Geometry check sheet. Reference: the model listing, model coordinates, mm. A direction names the side the tool comes from. Round coordinates to 2 decimals unless told otherwise and drop trailing zeros. Loops run counter-clockwise (first coordinate to the right, second up) from the corner with the lowest first, then second, coordinate; pieces in that order, holes last. Notation, with made-up numbers: M 34,15.25 L 61,15.25 A23 ccw 61,25.25 Z; hole C 38,0.25 d8. An arc over 180 degrees is marked long. Answer in a Markdown table with one row per item. Add a question column.
Autodesk Fusion 360 part; units mm, degrees
sketch "Skizze1" plane through (0, 0, 0) normal (0, 0, 1) x (1, 0, 0)
  circle A0 centre (0, 0) radius 7.55
  line L0 (20, -10) -> (-10, -10)
  line L1 (-10, -10) -> (-10, 53.5)
  line L2 (-10, 53.5) -> (20, 53.5)
  line L3 (20, 53.5) -> (20, -10)
  line L4 (0, 0) -> (0, -10)
  line L5 (0, -10) -> (-0.5, -10)
  line L6 (-0.5, -10) -> (0.5, -10)
  line L7 (0.5, -10) -> (0.5, -7.3)
  line L8 (0.5, -7.3) -> (-0.5, -7.3)
  line L9 (-0.5, -7.3) -> (-0.5, -10)
  line L10 (-18, 3.5) -> (-18, -3.5)
  line L11 (-18, 3.5) -> (-18.5, 3.5)
  line L12 (-18, -3.5) -> (-18.5, -3.5)
  line L13 (-18.5, -3.5) -> (-18.5, -10)
  line L14 (-18.5, -10) -> (-10, -10)
  line L15 (-18.5, 3.5) -> (-18.5, 8.5)
  line L16 (-18.5, 8.5) -> (-10, 8.5)
  line L17 (-10, 53.5) -> (-20, 53.5)
  line L18 (-20, 53.5) -> (-20, 8.5)
  line L19 (-20, 8.5) -> (-10, 8.5)
  line L20 (-10, 8.5) -> (-10, 53.5)
  dimension "d1" = 15.1
  dimension "d4" = 20
  dimension "d5" = 10
  dimension "d6" = 10
  dimension "d7" = 63.5
  dimension "d15" = 18
  dimension "d16" = 7
  dimension "d17" = 3.5
  dimension "d18" = 0.5
  dimension "d19" = 0.5
  dimension "d54" = 10
extrude "Extrusion1" add sketch "Skizze1" along normal blind 50 contours A0 L0 L1 L2 L3 L7 L9 L20 | L1 L10 L11 L12 L13 L14 L15 L16 L19 | L1 L16 L17 L18 L19 L20
sketch "Skizze2" plane through (20, 0, 0) normal (1, 0, 0) x (0, 1, 0)
  line L0 (-10, 0) -> (53.5, 0)
  line L1 (53.5, 0) -> (53.5, 50)
  line L2 (53.5, 50) -> (-10, 50)
  line L3 (-10, 50) -> (-10, 0)
  circle A0 centre (0, 25) radius 4.15
  circle A1 centre (30, 25) radius 11.75
  line L4 (14.5, 40.5) -> (45.5, 40.5)
  line L5 (45.5, 40.5) -> (45.5, 9.5)
  line L6 (45.5, 9.5) -> (14.5, 9.5)
  line L7 (14.5, 9.5) -> (14.5, 40.5)
  circle A2 centre (14.5, 40.5) radius 3.25
  circle A3 centre (45.5, 40.5) radius 3.25
  circle A4 centre (45.5, 9.5) radius 3.25
  circle A5 centre (14.5, 9.5) radius 3.25
  circle A6 centre (14.5, 40.5) radius 1.75
  circle A7 centre (45.5, 40.5) radius 1.75
  circle A8 centre (45.5, 9.5) radius 1.75
  circle A9 centre (14.5, 9.5) radius 1.75
  circle A10 centre (0, 7.5) radius 4.15
  circle A11 centre (0, 42.5) radius 4.15
  dimension "d10" = 8.3
  dimension "d11" = 10
  dimension "d42" = 25
  dimension "d55" = 30
  dimension "d56" = 25
  dimension "d57" = 23.5
  dimension "d58" = 31
  dimension "d59" = 31
  dimension "d60" = 15.5
  dimension "d61" = 15.5
  dimension "d62" = 6.5
  dimension "d63" = 3.5
  dimension "d78" = 10
  dimension "d80" = 10
  dimension "d81" = 17.5
  dimension "d82" = 17.5
extrude "Extrusion7" cut sketch "Skizze2" against normal blind 40 contours A1 | L4 L7 A6 | L4 L7 A6 | L4 L5 A7 | L4 L5 A7 | L6 L7 A9 | L6 L7 A9 | L5 L6 A8 | L5 L6 A8
extrude "Extrusion8" cut sketch "Skizze2" against normal blind 35 contours L4 L7 A2 A6 | L4 L7 A2 A6 | L4 L5 A3 A7 | L4 L5 A3 A7 | L6 L7 A5 A9 | L6 L7 A5 A9 | L5 L6 A4 A8 | L5 L6 A4 A8
extrude "Extrusion2" cut sketch "Skizze2" against normal blind 11 contours A0 | A10 | A11
sketch "Skizze3" plane through (0, 0, 50) normal (0, 0, 1) x (-1, 0, 0)
  line L0 (18, -3.5) -> (18, 3.5)
  line L1 (18, 3.5) -> (18.5, 3.5)
  line L2 (18.5, 3.5) -> (18.5, 10)
  line L3 (18.5, 10) -> (10, 10)
  line L4 (10, 10) -> (0.5, 10)
  line L5 (0.5, 10) -> (0.5, 7.5334)
  arc A0 (-0.5, 7.5334) -> (0.5, 7.5334) centre (0, 0) ccw
  line L6 (-0.5, 7.5334) -> (-0.5, 10)
  line L7 (-0.5, 10) -> (-20, 10)
  line L8 (-20, 10) -> (-20, -53.5)
  line L9 (-20, -53.5) -> (20, -53.5)
  line L10 (18.5, -8.5) -> (18.5, -3.5)
  line L11 (18.5, -3.5) -> (18, -3.5)
  line L12 (-20, -53.5) -> (10, -53.5)
  line L13 (10, -53.5) -> (10, -8.5)
  line L14 (-20, -8.5) -> (-20, -53.5)
  arc A1 (-10, -8.5) -> (10, -8.5) centre (0, 0) ccw
  line L15 (-10, -8.5) -> (-20, -8.5)
  line L16 (20, -53.5) -> (20, -8.5)
  line L17 (20, -8.5) -> (18.5, -8.5)
sketch "Skizze5" plane through (0, 53.5, 0) normal (0, 1, 0) x (-1, 0, 0)
  line L0 (-20, 50) -> (-20, 0)
  line L1 (-20, 0) -> (20, 0)
  line L2 (-20, 25) -> (-13, 25)
  line L3 (-13, 25) -> (-13, 29.75)
  line L4 (-13, 25) -> (-13, 20.25)
  circle A0 centre (-13, 29.75) radius 1.15
  circle A1 centre (-13, 20.25) radius 1.15
  line L5 (20, 50) -> (-20, 50)
  line L6 (20, 0) -> (20, 50)
  dimension "d23" = 7
  dimension "d24" = 4.75
  dimension "d25" = 2.3
  dimension "d26" = 2.3
extrude "Extrusion4" cut sketch "Skizze5" against normal blind 11 contours A0 | A1
sketch "Skizze6" plane through (-18.5, 0, 0) normal (-1, 0, 0) x (0, -1, 0)
  line L0 (-8.5, 0) -> (-3.5, 0)
  line L1 (-3.5, 0) -> (-3.5, 50)
  line L2 (-3.5, 50) -> (-8.5, 50)
  line L3 (-6, 50) -> (-6, 0)
  line L4 (6, 50) -> (6, 0)
  circle A0 centre (-6, 42.5) radius 1.5
  circle A1 centre (-6, 7.5) radius 1.5
  circle A2 centre (6, 7.5) radius 1.5
  circle A3 centre (6, 42.5) radius 1.5
  line L5 (3.5, 50) -> (10, 50)
  line L6 (3.5, 0) -> (10, 0)
  line L7 (-8.5, 50) -> (-8.5, 0)
  circle A4 centre (-6, 42.5) radius 3.25
  circle A5 centre (-6, 7.5) radius 3.25
  dimension "d29" = 12
  dimension "d30" = 3
  dimension "d31" = 3
  dimension "d32" = 3
  dimension "d33" = 3
  dimension "d35" = 7.5
  dimension "d36" = 7.5
  dimension "d37" = 7.5
  dimension "d38" = 7.5
  dimension "d73" = 6.5
  dimension "d74" = 6.5
extrude "Extrusion5" cut sketch "Skizze6" against normal blind 7 contours L3 A1 | L3 A1 | L3 A0 | L3 A0 | L4 A3 | L4 A2 | L4 A2 | L4 A3
sketch "Skizze9" plane through (0, 53.5, 0) normal (0, 1, 0) x (-1, 0, 0)
  circle A0 centre (-13, 29.75) radius 1.15
  circle A1 centre (-13, 20.25) radius 1.15
  line L0 (-20, 0) -> (20, 0)
  line L1 (20, 0) -> (20, 50)
  line L2 (20, 50) -> (-20, 50)
  line L3 (-20, 50) -> (-20, 0)
  line L4 (-20, 35) -> (-5, 35)
  line L5 (-5, 35) -> (-5, 15)
  line L6 (-5, 15) -> (-20, 15)
  line L7 (-20, 15) -> (-20, 35)
  line L8 (-20, 40.5) -> (-20, 9.5)
  point P0 (-20, 25)
  dimension "d68" = 15
  dimension "d69" = 20
  dimension "d70" = 10
extrude "Extrusion9" cut sketch "Skizze9" against normal blind 6 contours L3 L4 L5 L6 L7 L8
sketch "Skizze10" plane through (0, 0, 0) normal (0, 0, 1) x (1, 0, 0)
equation "d60 = ( 31 / 2 ) * 1 mm"
equation "d61 = ( 31 / 2 ) * 1 mm"
1) Cross-section at D-D, the plane z = 27. Record the boundary of the cut face in (x, y).
2) Go/stop test with flat-tipped pins: pin 1 (1.5 mm diameter, centred on y = -6, z = 8, fed in from -X); pin 2 (12 mm diameter, centred on x = 10, z = 21, fed in from +Y); pin 3 (5 mm diameter, centred on y = 24, z = 31.5, fed in from +X); pin 4 (1.1 mm diameter, centred on x = 13, z = 30, fed in from +Y). Record where each tip stops, or that it passes through.
3) Thickness scan on L1, parallel to Z at x = 7.5, y = 45.5; L2, parallel to Z at x = -15, y = -6; L3, parallel to X at y = 0, z = 40. Record the ranges inside material, lowest first. Write a range as [from, to].
4) Cross-section at A-A, the plane y = 30. Record the boundary of the cut face in (x, z).
5) Draft check along Z on faces 6 (the flat face through (12, 51, 15)), 7 (the flat face through (-18.5, 6, 25)), 8 (the flat face through (0, 22, 0)). Enter one of: +Z half, -Z half, draft (parallel to the pull), parting line (faces both ways), or undercut.
6) Cross-section at C-C, the plane x = -4.5. Record the boundary of the cut face in (y, z), plus the area to 3 significant figures.
7) Cross-section at B-B, the plane y = 45.5. Record the boundary of the cut face in (x, z).
8) Set-up check for faces 1 (the flat face through (13, 42.5, 20)), 2 (the cylindrical face through (2.745, 13.795, 37.327)), 3 (the flat face through (-11.5, -6, 43)), 4 (the flat face through (-0.5, -9, 25)), 5 (the cylindrical face through (-17.465, 47.117, 39.83)): record each of +Z, -Z, +X, -X, +Y, -Y from which the full face is reachable in a straight line by a thin tool's end or side.
Worked answers:
| question | item | result |
|---|---|---|
| 1 | outline | M -20,8.5 L -18.5,8.5 L -18.5,3.5 L -18,3.5 L -18,-3.5 L -18.5,-3.5 L -18.5,-10 L -0.5,-10 L -0.5,-7.53 A7.55 cw long 0.5,-7.53 L 0.5,-10 L 20,-10 L 20,-3.64 L 9,-3.64 L 9,3.64 L 20,3.64 L 20,18.42 L -20,18.42 Z; M -20,41.58 L 20,41.58 L 20,47.5 L 5,47.5 L 5,53.5 L -20,53.5 Z |
| 2 | pin 1 | stops at x = -11.5 |
| 2 | pin 2 | stops at y = 53.5 |
| 2 | pin 3 | passes through |
| 2 | pin 4 | stops at y = 42.5 |
| 3 | L1 | z = [0, 6.25], [12.75, 37.25], [43.75, 50] |
| 3 | L2 | z = [0, 6], [9, 41], [44, 50] |
| 3 | L3 | x = [-18, -7.55], [7.55, 9] |
| 4 | outline | M -20,0 L 20,0 L 20,13.25 L -20,13.25 Z; M -20,36.75 L 20,36.75 L 20,50 L -20,50 Z |
| 5 | face 6 | undercut |
| 5 | face 7 | draft |
| 5 | face 8 | -Z half |
| 6 | outline | M -10,0 L -6.06,0 L -6.06,50 L -10,50 Z; M 6.06,0 L 53.5,0 L 53.5,50 L 6.06,50 Z; hole C 14.5,9.5 d6.5; hole C 14.5,40.5 d6.5; hole C 30,25 d23.5; hole C 45.5,9.5 d6.5; hole C 45.5,40.5 d6.5 |
| 6 | area | 2,000 mm2 |
| 7 | outline | M -20,0 L 20,0 L 20,6.25 L -15,6.25 L -15,7.75 L -20,7.75 Z; M -20,11.25 L -15,11.25 L -15,12.75 L 20,12.75 L 20,37.25 L -15,37.25 L -15,38.75 L -20,38.75 Z; M -20,42.25 L -15,42.25 L -15,43.75 L 20,43.75 L 20,50 L -20,50 Z; hole C 13,20.25 d2.3; hole C 13,29.75 d2.3 |
| 8 | face 1 | +Y |
| 8 | face 2 | +X |
| 8 | face 3 | -X |
| 8 | face 4 | +Z, -Z, -Y |
| 8 | face 5 | +X, -X |
